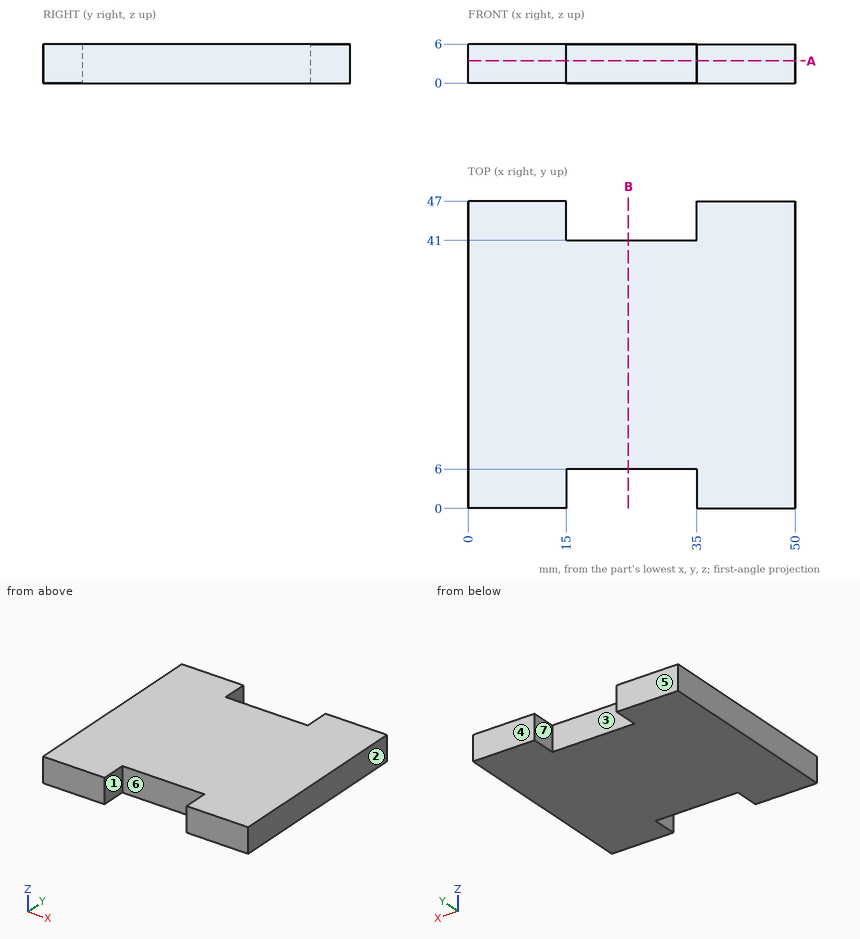
Could you check a few things on this drawing? It's one solid part, dimensions in mm from its lowest x, y, z. A direction names the side the tool comes from. Give positions to 0.01 mm unless a question says otherwise; leave off trailing zeros. Order: outer loops, then holes, each group sorted by start corner. A loop starts at its lowest first (then second) coordinate and runs counter-clockwise, first axis right, second up. Notation, with made-up numbers: (63, -16.5) - (95, -16.5) arc R18 cw to (95, 17.5) - close; hole circle Ø8 at (-20, -39.75). An arc over 180 degrees is marked (long way). Answer as a JSON object with one key per item and string values. Group by question number.
Item 1: Which directions (+Z, -Z, +X, -X, +Y, -Y) give clear straight access to the entire face, cutting with the end or side of a thin tool? Please do the marked faces 5, 6 and 7.
Item 2: For P1, Ø2, axis at x = 19.5, z = 1.5, coming from the -Y side, with a flat end and sliding along its axis, tell me the tip position at first contact or that it passes through.
Item 3: If we section it at A-A on z = 3.4: Please give me the cut outline in (x, y), and give its area (3 significant figures).
Item 4: If we section it at B-B on x = 24.5: Please give me the cut outline in (y, z).
Item 5: If we mould it in two halves opening along X, with no side actions, what happens to the marked faces 1, 2, 3 and 4? For each: pulls with the +X half, pulls with the -X half, needs draft (parallel to the pull), parting line crosses it, or undercut.
Item 6: Please list where these lines run through material, in increasing order: probe 1 along X at (y, z) = (42, 1.8); probe 2 along Y at (x, z) = (24, 1.55).
Result set:
{
 "1": {"face 5": "+Z, -Z, +X, -X, +Y", "face 6": "+Z, -Z, -Y", "face 7": "+Z, -Z, +Y"},
 "2": {"P1": "y = 6"},
 "3": {"outline": "(0, 0) - (15, 0) - (15, 6) - (35, 6) - (35, 0) - (50, 0) - (50, 47) - (35, 47) - (35, 41) - (15, 41) - (15, 47) - (0, 47) - close", "area": "2,110 mm²"},
 "4": {"outline": "(6, 0) - (41, 0) - (41, 6) - (6, 6) - close"},
 "5": {"face 1": "undercut", "face 2": "pulls with the +X half", "face 3": "undercut", "face 4": "needs draft"},
 "6": {"probe 1": "0 to 15, 35 to 50", "probe 2": "6 to 41"}
}
